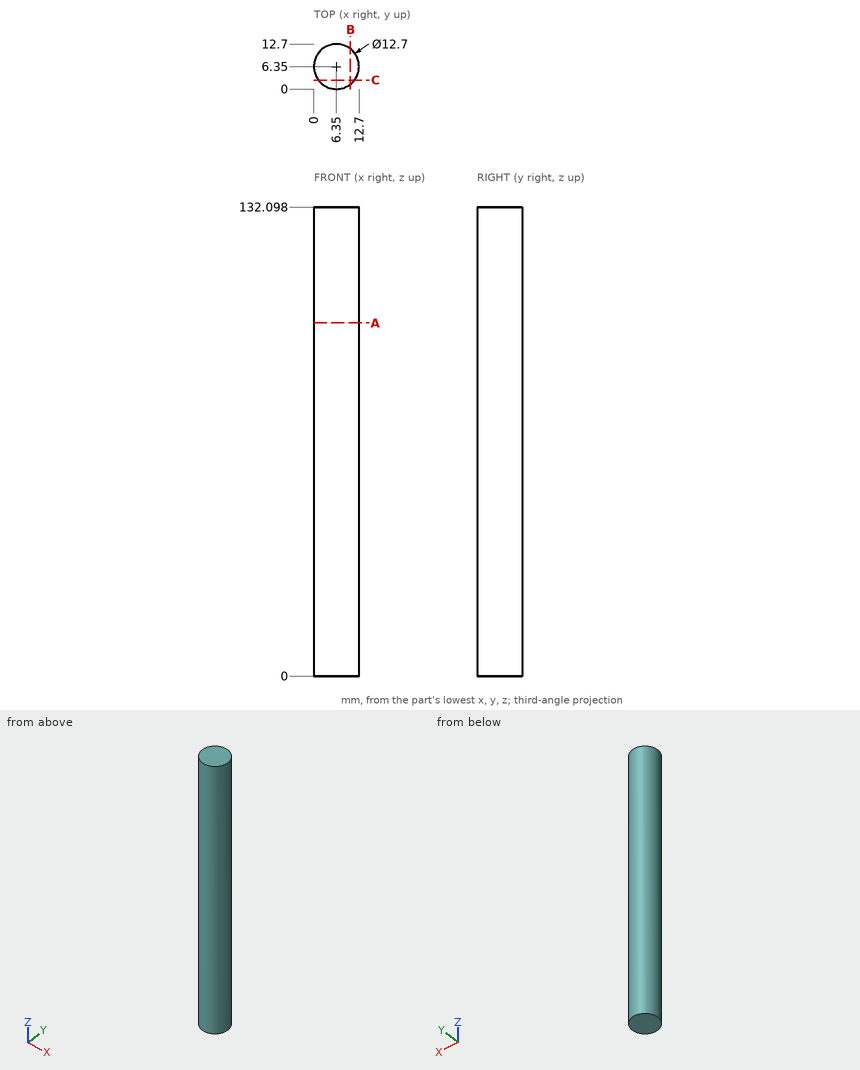
Answer from the drawing. Dimensions are ordinates in mm from the lowest x, y and z of the part. Round coordinates to 2 decimals unless told otherwise and drop trailing zeros. Write each loop counter-clockwise with the first axis right and the second up, starting at its lowest first coordinate (ties: lowest second). Pieces come first, ordered by that corner, then holes. Notation, with made-up numbers: (-30, 20) - (3, 20) arc R19 cw to (3, 48) - close; hole circle Ø7 at (4.5, 84.5). An arc over 180 degrees is marked (long way). Use a Markdown table: item, result.
(1) The part is cut by section A-A (z = 99.5). Write down the section's boundary in (x, y), then the cut area to 3 significant figures.
Reported:
| item | result |
|---|---|
| outline | circle Ø12.7 at (6.35, 6.35) |
| area | 127 mm2 |
(2) Straight lines are drawn through the part: line 1 along X through (y, z) = (6.5, 116.5); line 2 along Y through (x, z) = (6, 30); line 3 along Y through (x, z) = (10, 38). For each, find the intervals that lie inside material, in ascending order. Write a range as [from, to].
Reported:
| item | result |
|---|---|
| line 1 | [0, 12.7] |
| line 2 | [0.01, 12.69] |
| line 3 | [1.15, 11.55] |
(3) The part is cut by section C-C (y = 2.5). Write down the section's boundary in (x, z), then the cut area to 3 significant figures.
Reported:
| item | result |
|---|---|
| outline | (1.3, 0) - (11.4, 0) - (11.4, 132.1) - (1.3, 132.1) - close |
| area | 1,330 mm2 |
(4) The part is cut by section B-B (x = 10.25). Write down the section's boundary in (y, z).
Reported:
| item | result |
|---|---|
| outline | (1.34, 0) - (11.36, 0) - (11.36, 132.1) - (1.34, 132.1) - close |
(5) Each of these flat-tipped pins is pushed along its axis until it touches: pin 1 Ø1.5 at (x, z) = (2.5, 23.5) entering from -Y; pin 2 Ø5 at (x, z) = (1.5, 79.5) entering from -Y; pin 3 Ø1 at (x, z) = (7, 67) entering from +Y. Where does it stop, or does it pass through?
Reported:
| item | result |
|---|---|
| pin 1 | y = 0.81 |
| pin 2 | y = 0.45 |
| pin 3 | y = 12.7 |
